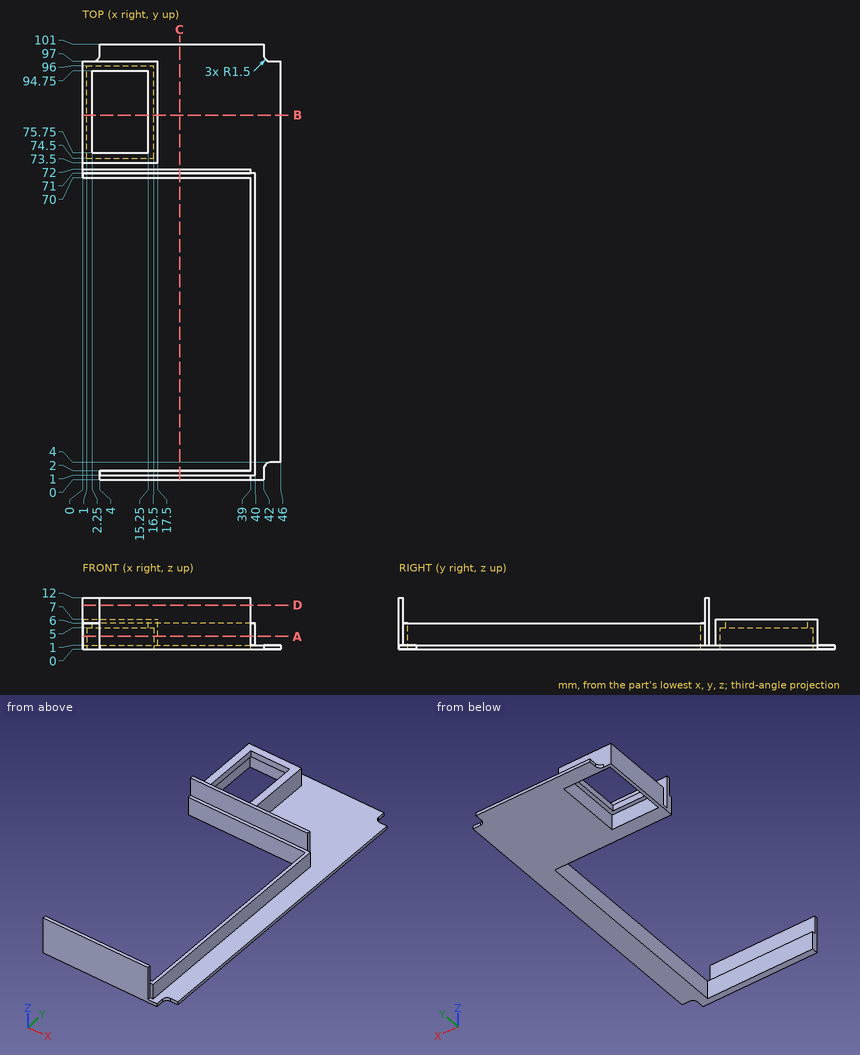
For this review, use the dimensioned drawing (mm, ordinates from the lowest corner) and the shaded views. Give positions to 0.01 mm unless a question says otherwise; leave off trailing zeros. Write each loop counter-clockwise with the first axis right and the second up, starting at its lowest first coordinate (ties: lowest second). Pieces come first, ordered by that corner, then holes. Notation, with made-up numbers: M -0.75,40 L 6.25,40 A11 ccw 6.25,48 Z; hole C 80,4.25 d3. An arc over 180 degrees is marked long. Answer as a JSON object with one key per item and string values. Group by question number.
Item 1: Consider section C-C on x = 22.5. Write out the cut boundary in (y, z).
Item 2: Consider section D-D on z = 10.25. Write out the cut boundary in (x, y).
Item 3: Consider section B-B on y = 84.5. Write out the cut boundary in (x, z).
Item 4: For pin 1 Ø5.5 at (x, z) = (19, 6.5) entering from +Y; pin 2 Ø2.5 at (y, z) = (84, 3.5) entering from +X; pin 3 Ø5.5 at (y, z) = (84, 3.5) entering from -X; pin 4 Ø1.1 at (y, z) = (0.5, 6) entering from +X, all flat-tipped, find the tip position at first contact; note any pin that passes through.
Item 5: Consider section A-A on z = 3. Write out the cut boundary in (x, y).
Item 6: For probe 1 along Y at (x, z) = (11.5, 3); probe 2 along Y at (x, z) = (12.5, 5.5); probe 3 along Y at (x, z) = (20, 7), list the stretches that pass through material, from the lowest coordinate up. Write a range as [from, to].
Check result:
{
 "1": {"outline": "M 0,0 L 2,0 L 2,6 L 1,6 L 1,12 L 0,12 Z; M 70,0 L 101,0 L 101,1 L 72,1 L 72,12 L 71,12 L 71,6 L 70,6 Z"},
 "2": {"outline": "M 0,71 L 39,71 L 39,72 L 0,72 Z; M 4,0 L 39,0 L 39,1 L 4,1 Z"},
 "3": {"outline": "M 0,0 L 1,0 L 1,5 L 2.25,5 L 2.25,7 L 0,7 Z; M 15.25,5 L 16.5,5 L 16.5,0 L 46,0 L 46,1 L 17.5,1 L 17.5,7 L 15.25,7 Z"},
 "4": {"pin 1": "stops at y = 97", "pin 2": "stops at x = 17.5", "pin 3": "stops at x = 0", "pin 4": "stops at x = 40"},
 "5": {"outline": "M 0,70 L 39,70 L 39,2 L 4,2 L 4,0 L 39,0 L 39,1 L 40,1 L 40,71 L 39,71 L 39,72 L 0,72 Z; M 0,73.5 L 17.5,73.5 L 17.5,97 L 0,97 Z; hole M 1,74.5 L 16.5,74.5 L 16.5,96 L 1,96 Z"},
 "6": {"probe 1": "y = [0, 2], [70, 72], [73.5, 74.5], [96, 97]", "probe 2": "y = [0, 2], [70, 72], [73.5, 75.75], [94.75, 97]", "probe 3": "y = [0, 1], [71, 72]"}
}
